Can you work these out from the model? Positions are in its coordinate system, mm. Coordinates: 2 decimals unless noted, no trailing zeros. Loops run counter-clockwise (first coordinate to the right, second up) from the corner with the lowest first, then second, coordinate; pieces in that order, holes last. Notation, with made-up numbers: (15.25, 24) -> (36.25, 24) arc R33 ccw to (36.25, 52) -> close; hole circle Ø4 at (69.25, 9.25). An arc over 180 degrees is marked (long way). Put each result on its own line as item: value. Start each with the question number.
Item 1: We'd pull the mould along Z, two halves only. Please class faces 1 (the flat face through (-4, 27.365, 22)), 2 (the cylindrical face through (16.89, 13.53, -8.78)), 3 (the cylindrical face through (24.397, 13.533, -12.69)): pulls with the +Z half, pulls with the -Z half, needs draft (parallel to the pull), parting line crosses it, or undercut.
Item 2: If we section it at D-D on y = 25.25: Please give me the cut outline in (x, z), plus the area to 3 significant figures.
Item 3: If we section it at C-C on y = 14.25: Please give me the cut outline in (x, z), plus the area to 3 significant figures.
Item 4: Will these pins go through, and if not, where does the flat tip stop? P1, Ø8, axis at x = 15, y = 18.5, coming from the +Z side; P2, Ø5, axis at x = -16, y = 14.5, coming from the -Z side; P3, Ø10, axis at y = 9, z = 8.5, coming from the -X side.
Item 5: If we section it at A-A on x = 0: Please give me the cut outline in (y, z).
Item 6: Please list where these lines run through material, in increasing order: L1, parallel to X at y = 18, z = 0; L2, parallel to Z at x = 13, y = 2.75; L3, parallel to Z at x = -9.5, y = 16. Write a range as from..to.
Item 7: If we section it at B-B on z = 0: Please give me the cut outline in (x, y).
```python
from build123d import *

# Parameters (mm, degrees)
SKETCH1_R           = 27.5
BOSS_EXTRUDE1_DEPTH = 27.364676
SKETCH2_R           = 19.033814865
CUT_EXTRUDE1_DEPTH  = 48.553396226
CHAMFER1_SIZE       = 3.003375


with BuildPart() as part:
    # Sketch1 → Boss-Extrude1 (new body)
    with BuildSketch(Plane(origin=(0, 0, 0), x_dir=(1, 0, 0), z_dir=(0, 1, 0))):
        with Locations(Location((0, 0, 0), (0, 0, 90))):
            Circle(SKETCH1_R)
    extrude(amount=BOSS_EXTRUDE1_DEPTH)

    # Sketch2 → Cut-Extrude1 (cut, through all)
    with BuildSketch(Plane(origin=(0, 0, 0), x_dir=(1, 0, 0), z_dir=(0, 1, 0))):
        with Locations(Location((0, 0, 0), (0, 0, 90))):
            Circle(SKETCH2_R)
    extrude(amount=CUT_EXTRUDE1_DEPTH, mode=Mode.SUBTRACT)

    # Chamfer1
    chamfer1_edges = [part.edges().sort_by_distance(p)[0] for p in [
        (0, 0, 27.5),
        (0, 27.364676, 27.5),
        (0, 0, 19.033814865),
        (0, 27.364676, 19.033814865),
    ]]
    chamfer(chamfer1_edges, length=CHAMFER1_SIZE)


solid = part.part
```
Solutions:
1. face 1: needs draft
1. face 2: undercut
1. face 3: parting line crosses it
2. outline: circle Ø53.22 at (0, 0); hole circle Ø39.85 at (0, 0)
2. area: 978 mm^2
3. outline: circle Ø55 at (0, 0); hole circle Ø38.07 at (0, 0)
3. area: 1,240 mm^2
4. P1: z = 25.2
4. P2: z = -23.96
4. P3: x = -27.28
5. outline: (0, -24.5) -> (3, -27.5) -> (24.36, -27.5) -> (27.36, -24.5) -> (27.36, -22.04) -> (24.36, -19.03) -> (3, -19.03) -> (0, -22.04) -> close; (0, 22.04) -> (3, 19.03) -> (24.36, 19.03) -> (27.36, 22.04) -> (27.36, 24.5) -> (24.36, 27.5) -> (3, 27.5) -> (0, 24.5) -> close
6. L1: -27.5..-19.03, 19.03..27.5
6. L2: -23.95..-14.25, 14.25..23.95
6. L3: -25.81..-16.49, 16.49..25.81
7. outline: (-27.5, 3) -> (-24.5, 0) -> (-22.04, 0) -> (-19.03, 3) -> (-19.03, 24.36) -> (-22.04, 27.36) -> (-24.5, 27.36) -> (-27.5, 24.36) -> close; (19.03, 3) -> (22.04, 0) -> (24.5, 0) -> (27.5, 3) -> (27.5, 24.36) -> (24.5, 27.36) -> (22.04, 27.36) -> (19.03, 24.36) -> close
